Part print with two shaded views. Sizes in mm from the minimum x, y, z corner. Give positions to 0.01 mm unless a question says otherwise; leave off trailing zeros. Loops run counter-clockwise (first coordinate to the right, second up) from the corner with the lowest first, then second, coordinate; pieces in that order, holes last. Notation, with made-up numbers: M -14.75,-13 L 33.25,-13 A24 cw 33.25,0 Z; hole C 62.25,43.25 d5. An arc over 180 degrees is marked long. Answer in a Markdown table with one row per item.
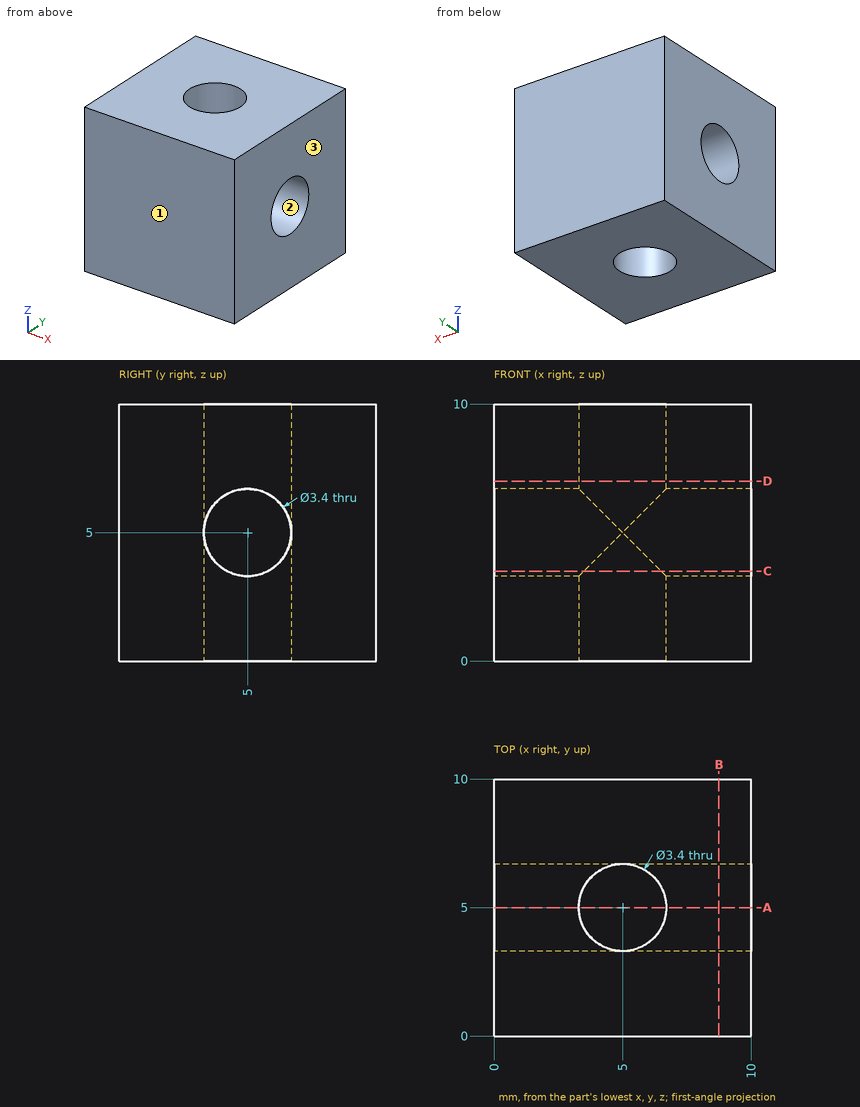
Q1. Saw through at B-B (x = 8.75). Give the cut face in (y, z), and give its area (3 significant figures).
Reported:
| item | result |
|---|---|
| outline | M 0,0 L 10,0 L 10,10 L 0,10 Z; hole C 5,5 d3.4 |
| area | 90.9 mm² |
Q2. Saw through at C-C (z = 3.5). Give the cut face in (x, y), and give its area (3 significant figures).
Reported:
| item | result |
|---|---|
| outline | M 0,0 L 10,0 L 10,4.2 L 6.5,4.2 A1.7 cw 3.5,4.2 L 0,4.2 Z; M 0,5.8 L 3.5,5.8 A1.7 cw 6.5,5.8 L 10,5.8 L 10,10 L 0,10 Z |
| area | 80.2 mm² |
Q3. Drop a flat-ended pin along its axis: pin 1 (2 mm diameter, centred on x = 5, y = 5, fed in from -Z) (1 decimal). Give the stop position or say it passes through.
Reported:
| item | result |
|---|---|
| pin 1 | through |
Q4. Saw through at A-A (y = 5). Give the cut face in (x, z), and give its area (3 significant figures).
Reported:
| item | result |
|---|---|
| outline | M 0,0 L 3.3,0 L 3.3,3.3 L 0,3.3 Z; M 0,6.7 L 3.3,6.7 L 3.3,10 L 0,10 Z; M 6.7,0 L 10,0 L 10,3.3 L 6.7,3.3 Z; M 6.7,6.7 L 10,6.7 L 10,10 L 6.7,10 Z |
| area | 43.6 mm² |
Q5. Probe probe 1 along Z at (x, y) = (2.75, 5). List the from-to ranges inside material, lowest first.
Reported:
| item | result |
|---|---|
| probe 1 | 0 to 3.3, 6.7 to 10 |
Q6. Mould opens along Y. For the marked faces 1, 2 and 3 say: released by +Y, released by -Y, zero draft, split by the parting line, or undercut.
Reported:
| item | result |
|---|---|
| face 1 | released by -Y |
| face 2 | undercut |
| face 3 | zero draft |
